from build123d import *

# Parameters (mm, degrees)
MODEL_R             = 4
MODEL_W             = 5.350001156
MODEL_H             = 4.999999889
MODEL_W_2           = 5.349997431
BOSS_EXTRUDE1_DEPTH = 5.35


with BuildPart() as part:
    # Model → Boss-Extrude1 (new body)
    with BuildSketch(Plane.XY):
        Polygon((70.000000298, 5.350000225), (70.000000298, 19.350000657), (0, 19.350000657), (0, 5.350000225), (13.99999857, 5.350000225), (13.99999857, 0), (28.000000864, 0), (28.000000864, 5.350000225), (41.999999434, 5.350000225), (41.999999434, 0), (55.999999866, 0), (55.999999866, 5.350000225), align=None)
        with Locations((7.000000298, 12.350000225)):
            Circle(MODEL_R, mode=Mode.SUBTRACT)
        with Locations((63.000000298, 12.350000225)):
            Circle(MODEL_R, mode=Mode.SUBTRACT)
        with Locations((47.675000504, 12.349999976)):
            Rectangle(MODEL_W, MODEL_H, mode=Mode.SUBTRACT)
        with Locations((22.324999795, 12.349999976)):
            Rectangle(MODEL_W_2, MODEL_H, mode=Mode.SUBTRACT)
        Polygon((41.350852698, 12.350000441), (38.175426424, 17.850000411), (31.824573874, 17.850000411), (28.6491476, 12.350000441), (31.824573874, 6.850000238), (38.175426424, 6.850000238), align=None, mode=Mode.SUBTRACT)
    extrude(amount=BOSS_EXTRUDE1_DEPTH)


solid = part.part
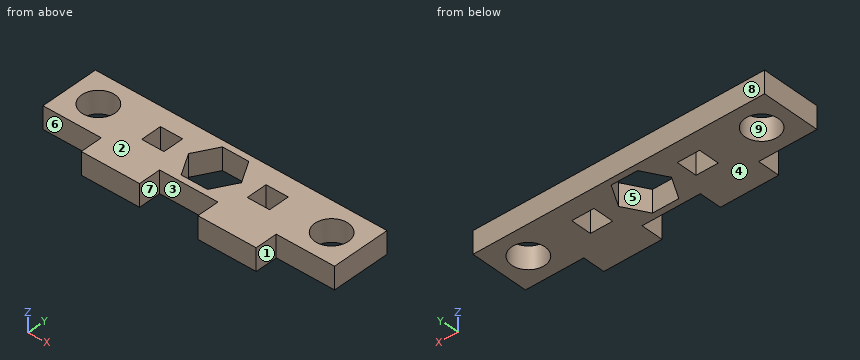
Input: part model. Units: mm. Frame: model coordinates. Face numbers are marked on the shaded views. A direction names the side the tool comes from. Coordinates: 2 decimals unless noted, no trailing zeros. Loops run counter-clockwise (first coordinate to the right, second up) from the corner with the lowest first, then second, coordinate; pieces in that order, holes last.
Q1. Set-up query: the marked faces 1, 2, 3, 4 and 5. Return all of +Z, -Z, +X, -X, +Y, -Y with unobstructed straight access to the full face (end or side cutting, diameter ignored); none if empty.
Q2. Cut plane C-C (x = 7). Output: boundary loops of the cut face in (y, z), then the cut area to 3 significant figures.
Q3. Cut plane D-D (y = 11.5). Output: boundary loops of the cut face in (x, z), then the cut area to 3 significant figures.
Q4. Material intervals for line 1 (X direction, y = 5.25, z = 0.2); line 2 (Y direction, x = 23, z = 3.75); line 3 (Y direction, x = 7, z = 2.45), sorted ascending.
Q5. Cut plane B-B (z = 3.2). Output: boundary loops of the cut face in (x, y).
Q6. Contact query for flat-ended pins moving along their axis: pin 1 (2.5 mm diameter, centred on x = 35.5, z = 1.5, fed in from -Y); pin 2 (1.6 mm diameter, centred on y = 3, z = 2, fed in from +X); pin 3 (1.6 mm diameter, centred on y = 1.5, z = 3.5, fed in from -X). Output: stop coordinate, or through.
Q7. Draft query along Y for the marked faces 6, 7, 8 and 9. Return one class per face: +Y half, -Y half, draft (parallel to the pull), parting line (faces both ways), or undercut.
Q8. Cut plane A-A (y = 4.25). Output: boundary loops of the cut face in (x, z), then the cut area to 3 significant figures.
Working result:
1. face 1: +Z, -Z, +X, -Y
1. face 2: +Z, +X, -X, +Y, -Y
1. face 3: +Z, -Z, -Y
1. face 4: -Z, +X, -X, +Y, -Y
1. face 5: +Z, -Z
2. outline: (5.35, 0) - (8.35, 0) - (8.35, 5.35) - (5.35, 5.35) - close; (16.35, 0) - (19.35, 0) - (19.35, 5.35) - (16.35, 5.35) - close
2. area: 32.1 mm2
3. outline: (0, 0) - (3.09, 0) - (3.09, 5.35) - (0, 5.35) - close; (10.91, 0) - (19.65, 0) - (19.65, 5.35) - (10.91, 5.35) - close; (25, 0) - (29.14, 0) - (29.14, 5.35) - (25, 5.35) - close; (40.86, 0) - (45, 0) - (45, 5.35) - (40.86, 5.35) - close; (50.35, 0) - (59.09, 0) - (59.09, 5.35) - (50.35, 5.35) - close; (66.91, 0) - (70, 0) - (70, 5.35) - (66.91, 5.35) - close
3. area: 171 mm2
4. line 1: x = 14 to 28, 42 to 56
4. line 2: y = 0 to 9.85, 14.85 to 19.35
4. line 3: y = 5.35 to 8.35, 16.35 to 19.35
5. outline: (0, 5.35) - (14, 5.35) - (14, 0) - (28, 0) - (28, 5.35) - (42, 5.35) - (42, 0) - (56, 0) - (56, 5.35) - (70, 5.35) - (70, 19.35) - (0, 19.35) - close; hole circle Ø8 at (7, 12.35); hole (19.65, 9.85) - (25, 9.85) - (25, 14.85) - (19.65, 14.85) - close; hole (28.65, 12.35) - (31.82, 6.85) - (38.18, 6.85) - (41.35, 12.35) - (38.18, 17.85) - (31.82, 17.85) - close; hole (45, 9.85) - (50.35, 9.85) - (50.35, 14.85) - (45, 14.85) - close; hole circle Ø8 at (63, 12.35)
6. pin 1: stops at y = 5.35
6. pin 2: stops at x = 56
6. pin 3: stops at x = 14
7. face 6: -Y half
7. face 7: draft
7. face 8: +Y half
7. face 9: undercut
8. outline: (14, 0) - (28, 0) - (28, 5.35) - (14, 5.35) - close; (42, 0) - (56, 0) - (56, 5.35) - (42, 5.35) - close
8. area: 150 mm2
